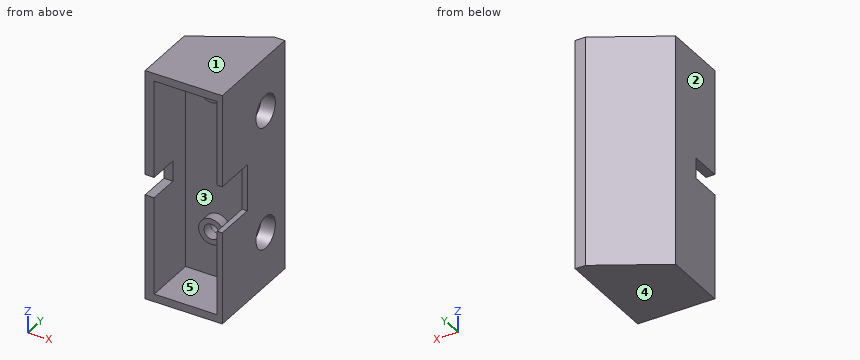
from build123d import *

# Parameters (mm, degrees)
PAD_DEPTH       = 22.5
SKETCH001_R     = 1.4
POCKET_DEPTH    = 13
SKETCH002_R     = 3.1
POCKET001_DEPTH = 2.8
SKETCH004_W     = 12.25
SKETCH004_H     = 42
POCKET002_DEPTH = 10
SKETCH010_R     = 2.5
SKETCH010_R_2   = 1.391107
SKETCH010_R_3   = 1.47119
PAD001_DEPTH    = 2
SKETCH006_W     = 12.042882
SKETCH006_H     = 4
POCKET003_DEPTH = 15.001
SKETCH011_W     = 13.213881
SKETCH011_H     = 9.078228
POCKET004_DEPTH = 5


with BuildPart() as part:
    # Sketch → Pad (new body, symmetric)
    with BuildSketch(Plane.XY):
        Polygon((0, 0), (-15, 0), (-15, 12.494447), (-2, 20), (0, 20), align=None)
    extrude(amount=PAD_DEPTH, both=True)

    # Sketch001 (on Face1 of Pad) → Pocket (cut)
    with BuildSketch(Plane.XZ):
        with Locations((-7, 17)):
            Circle(SKETCH001_R)
        with Locations((-7, -11)):
            Circle(SKETCH001_R)
    extrude(amount=-POCKET_DEPTH, mode=Mode.SUBTRACT)

    # Sketch002 → Pocket001 (cut)
    with BuildSketch(Plane.YZ):
        with Locations((13.88237, 12)):
            Circle(SKETCH002_R)
        with Locations((13.88237, -12)):
            Circle(SKETCH002_R)
    extrude(amount=-POCKET001_DEPTH, mode=Mode.SUBTRACT)

    # Sketch004 → Pocket002 (cut)
    with BuildSketch(Plane.XZ):
        with Locations((-7.125, 0)):
            Rectangle(SKETCH004_W, SKETCH004_H)
    extrude(amount=-POCKET002_DEPTH, mode=Mode.SUBTRACT)

    # Sketch010 (on Face14 of Pocket002) → Pad001 (join)
    with BuildSketch(Plane.XZ.offset(-10)):
        with Locations((-7.014447, 16.981703)):
            Circle(SKETCH010_R)
        with Locations((-7.014447, 16.981703)):
            Circle(SKETCH010_R_2, mode=Mode.SUBTRACT)
        with Locations((-6.967297, -10.977527)):
            Circle(SKETCH010_R)
        with Locations((-6.967297, -10.977527)):
            Circle(SKETCH010_R_3, mode=Mode.SUBTRACT)
    extrude(amount=PAD001_DEPTH)

    # Sketch006 → Pocket003 (cut, through all)
    with BuildSketch(Plane(origin=(-15, 0, 0), x_dir=(0, -1, 0), z_dir=(-1, 0, 0))):
        with Locations((0.021441, 0)):
            Rectangle(SKETCH006_W, SKETCH006_H)
    extrude(amount=-POCKET003_DEPTH, mode=Mode.SUBTRACT)

    # Sketch011 (on Face9 of Pocket003) → Pocket004 (cut)
    with BuildSketch(Plane.YZ):
        with Locations((1.39306, 0)):
            Rectangle(SKETCH011_W, SKETCH011_H)
    extrude(amount=-POCKET004_DEPTH, mode=Mode.SUBTRACT)


solid = part.part
Part model, mm, in its own coordinate system. Face numbers are marked on the shaded views. A direction names the side the tool comes from. Coordinates: 2 decimals unless noted, no trailing zeros. Order: outer loops, then holes, each group sorted by start corner. A loop starts at its lowest first (then second) coordinate and runs counter-clockwise, first axis right, second up.
(1) Tool access for the marked faces 4 and 5: list every direction of +Z, -Z, +X, -X, +Y, -Y with a clear straight run to the whole face (end or side of a thin tool).
Check sheet entries:
face 4: -Z, +X, -X, +Y, -Y
face 5: -Y
(2) Pin check, flat tips, straight feed: pin 1 Ø0.8 at (x, z) = (-6.5, 17.5) entering from -Y; pin 2 Ø3 at (x, z) = (-6.5, -11) entering from -Y; pin 3 Ø2 at (x, z) = (-13, 9) entering from +Y. Stop position of each tip, or through.
Check sheet entries:
pin 1: stops at y = 13
pin 2: stops at y = 8
pin 3: stops at y = 14.23
(3) Slice it at B-B, the plane z = 20.5. Write the cut outline in (x, y).
Check sheet entries:
outline: (-15, 0) - (-13.25, 0) - (-13.25, 10) - (-1, 10) - (-1, 0) - (0, 0) - (0, 20) - (-2, 20) - (-15, 12.49) - close
(4) Slice it at C-C, the plane y = 9.25. Write the cut outline in (x, z).
Check sheet entries:
outline: (-15, -22.5) - (0, -22.5) - (0, 22.5) - (-15, 22.5) - close; circle Ø5 at (-7.01, 16.98); circle Ø5 at (-6.97, -10.98); hole (-13.25, -21) - (-1, -21) - (-1, 21) - (-13.25, 21) - close; hole circle Ø2.94 at (-6.97, -10.98); hole circle Ø2.78 at (-7.01, 16.98)
(5) Slice it at A-A, the plane y = 3.25. Write the cut outline in (x, z), and give its area (3 significant figures).
Check sheet entries:
outline: (-15, -22.5) - (0, -22.5) - (0, -4.54) - (-1, -4.54) - (-1, -21) - (-13.25, -21) - (-13.25, -2) - (-15, -2) - close; (-15, 2) - (-13.25, 2) - (-13.25, 21) - (-1, 21) - (-1, 4.54) - (0, 4.54) - (0, 22.5) - (-15, 22.5) - close
area: 144 mm2
(6) Pull direction Z, two halves, no side cores. Call the marked faces 1, 2 and 3: pulls with the +Z half, pulls with the -Z half, needs draft (parallel to the pull), parting line crosses it, or undercut.
Check sheet entries:
face 1: pulls with the +Z half
face 2: needs draft
face 3: undercut
(7) Probe L1, parallel to X at y = 9.25, z = -7.5; L2, parallel to Z at x = -3.5, y = 6.25; L3, parallel to X at y = 6.25, z = -1. List the from-to ranges inside material, lowest first.
Check sheet entries:
L1: x = -15 to -13.25, -1 to 0
L2: z = -22.5 to -21, 21 to 22.5
L3: x = -15 to -13.25
